from build123d import *

# Parameters (mm, degrees)
SKETCH1_W                    = 304.8
SKETCH1_H                    = 50.8
BOSS_EXTRUDE1_DEPTH          = 4.064
F_1_8_0_125_DIAMETER_HOLE1_D = 3.175
SKETCH4_W                    = 127
SKETCH4_H                    = 50.8
CUT_EXTRUDE1_DEPTH           = 5.064


with BuildPart() as part:
    # Sketch1 → Boss-Extrude1 (new body)
    with BuildSketch(Plane(origin=(0, 0, 0), x_dir=(1, 0, 0), z_dir=(0, 1, 0))):
        with Locations((152.4, 25.4)):
            Rectangle(SKETCH1_W, SKETCH1_H)
    extrude(amount=BOSS_EXTRUDE1_DEPTH)

    # 1/8 (0.125) Diameter Hole1 (through all)
    with Locations(Plane(origin=(0, 4.064, 0), x_dir=(1, 0, 0), z_dir=(0, 1, 0))):
        with Locations((12.7, 12.7), (38.1, 38.1), (12.7, 38.1), (38.1, 12.7), (139.7, 12.7), (165.1, 38.1), (139.7, 38.1), (165.1, 12.7)):
            Hole(F_1_8_0_125_DIAMETER_HOLE1_D / 2)

    # Sketch4 → Cut-Extrude1 (cut, through all)
    with BuildSketch(Plane(origin=(0, 4.064, 0), x_dir=(1, 0, 0), z_dir=(0, 1, 0))):
        with Locations((241.3, 25.4)):
            Rectangle(SKETCH4_W, SKETCH4_H)
    extrude(amount=-CUT_EXTRUDE1_DEPTH, mode=Mode.SUBTRACT)


solid = part.part
Could you check a few things on this model? Use its own coordinates, in mm. Coordinates: 2 decimals unless noted, no trailing zeros. Loops run counter-clockwise (first coordinate to the right, second up) from the corner with the lowest first, then second, coordinate; pieces in that order, holes last.
1. I need wall thicknesses on L1, parallel to Z at x = 38.1, y = 2.2; L2, parallel to X at y = 1.4, z = -38.1; L3, parallel to X at y = 3.35, z = -39.5. Which ranges of each line are inside material? Lowest first, please.
2. Imagine slicing it at B-B (x = 139.7). Please give me the cut outline in (y, z), and give its area (3 significant figures).
3. For P1, Ø1.9, axis at x = 165.1, z = -12.7, coming from the -Y side, with a flat end and sliding along its axis, tell me the tip position at first contact or that it passes through.
4. Imagine slicing it at A-A (z = -38.1). Please give me the cut outline in (x, y).
5. We'd pull the mould along Z, two halves only. Please class faces 1 (the face through (166.27, 2.004, -13.773)), 2 (the face through (88, 2, 0)), 3 (the face through (36.586, 2.004, -13.177)), 4 (the face through (177.8, 2, -25)): released by +Z, released by -Z, zero draft, split by the parting line, or undercut.
Computed values:
1. L1: z = -50.8 to -39.69, -36.51 to -14.29, -11.11 to 0
1. L2: x = 0 to 11.11, 14.29 to 36.51, 39.69 to 138.11, 141.29 to 163.51, 166.69 to 177.8
1. L3: x = 0 to 11.95, 13.45 to 37.35, 38.85 to 138.95, 140.45 to 164.35, 165.85 to 177.8
2. outline: (0, -50.8) - (4.06, -50.8) - (4.06, -39.69) - (0, -39.69) - close; (0, -36.51) - (4.06, -36.51) - (4.06, -14.29) - (0, -14.29) - close; (0, -11.11) - (4.06, -11.11) - (4.06, 0) - (0, 0) - close
2. area: 181 mm2
3. P1: passes through
4. outline: (0, 0) - (11.11, 0) - (11.11, 4.06) - (0, 4.06) - close; (14.29, 0) - (36.51, 0) - (36.51, 4.06) - (14.29, 4.06) - close; (39.69, 0) - (138.11, 0) - (138.11, 4.06) - (39.69, 4.06) - close; (141.29, 0) - (163.51, 0) - (163.51, 4.06) - (141.29, 4.06) - close; (166.69, 0) - (177.8, 0) - (177.8, 4.06) - (166.69, 4.06) - close
5. face 1: undercut
5. face 2: released by +Z
5. face 3: undercut
5. face 4: zero draft
